```python
from build123d import *

# Parameters (mm, degrees)
CYLINDER026_R     = 1.5
CYLINDER026_DEPTH = 10
CYLINDER025_R     = 1.5
CYLINDER025_DEPTH = 10
CYLINDER024_R     = 1.5
CYLINDER024_DEPTH = 10
CYLINDER027_R     = 1.5
CYLINDER027_DEPTH = 10
BOX022_W          = 15.4
BOX022_H          = 47
BOX022_DEPTH      = 75.8
BOX021_W          = 17.6
BOX021_H          = 51.4
BOX021_DEPTH      = 78


with BuildPart() as obj1:
    # Cylinder026 → Cylinder026 (new body)
    with BuildSketch(Plane(origin=(50, 64.5, 56), x_dir=(0, 0, -1), z_dir=(1, 0, 0))):
        Circle(CYLINDER026_R)
    extrude(amount=CYLINDER026_DEPTH)


with BuildPart() as obj2:
    # Cylinder025 → Cylinder025 (new body)
    with BuildSketch(Plane(origin=(50, 29.5, 50), x_dir=(0, 0, -1), z_dir=(1, 0, 0))):
        Circle(CYLINDER025_R)
    extrude(amount=CYLINDER025_DEPTH)


with BuildPart() as obj3:
    # Cylinder024 → Cylinder024 (new body)
    with BuildSketch(Plane(origin=(50, 29.5, 56), x_dir=(0, 0, -1), z_dir=(1, 0, 0))):
        Circle(CYLINDER024_R)
    extrude(amount=CYLINDER024_DEPTH)


with BuildPart() as obj4:
    # Cylinder027 → Cylinder027 (new body)
    with BuildSketch(Plane(origin=(50, 64.5, 50), x_dir=(0, 0, -1), z_dir=(1, 0, 0))):
        Circle(CYLINDER027_R)
    extrude(amount=CYLINDER027_DEPTH)

    # Fusion015: union obj1, obj2, obj3
    add(obj1.part)
    add(obj2.part)
    add(obj3.part)


with BuildPart() as obj5:
    # Box022 → Box022 (new body)
    with BuildSketch(Plane(origin=(2.2, 2.2, 2.2), x_dir=(1, 0, 0), z_dir=(0, 0, 1))):
        with Locations((7.7, 23.5)):
            Rectangle(BOX022_W, BOX022_H)
    extrude(amount=BOX022_DEPTH)


with BuildPart() as obj6:
    # Box021 → Box021 (new body)
    with BuildSketch(Plane.XY):
        with Locations((8.8, 25.7)):
            Rectangle(BOX021_W, BOX021_H)
    extrude(amount=BOX021_DEPTH)

    # Cut022: cut obj5
    add(obj5.part, mode=Mode.SUBTRACT)


with BuildPart() as obj6_1:
    # Cut022 placement: moved
    add(obj6.part.moved(Location((50.2, 21.3, 41.8))))

    # Cut029: cut obj4
    add(obj4.part, mode=Mode.SUBTRACT)


solid = obj6_1.part
```
For this review, take the finished solid that the model builds, in its own axes (mm). A direction names the side the tool comes from. Round coordinates to 2 decimals unless told otherwise and drop trailing zeros. Write each loop counter-clockwise with the first axis right and the second up, starting at its lowest first coordinate (ties: lowest second). Pieces come first, ordered by that corner, then holes. Notation, with made-up numbers: (-26, 88.25) -> (14, 88.25) arc R9 cw to (14, 94.25) -> close; hole circle Ø6 at (46, -19). An arc over 180 degrees is marked (long way). One line per question, with ' | ' between items. Start each with the question number.
(1) Add section A-A, the plane y = 29.5. Write out the cut boundary in (x, z).
(2) For line 1 along Y through (x, z) = (51.6, 56); line 2 along Z through (x, y) = (51.65, 29.5); line 3 along Y through (x, z) = (61.75, 113), list the stretches that pass through material, from the lowest coordinate up. Write a range as from..to.
(3) Add section B-B, the plane z = 50. Write out the cut boundary in (x, y), plus the area to 3 significant figures.
(4) Add section C-C, the plane x = 56.25. Write out the cut boundary in (y, z).
(5) Tool access review of faces 4 (the face through (60, 47, 44)), 5 (the face through (59, 21.3, 80)): name each direction out of +Z, -Z, +X, -X, +Y, -Y from which nothing blocks a thin tool from reaching the whole face with its end or side.
(6) Add section D-D, the plane y = 42. Write out the cut boundary in (x, z), plus the area to 3 significant figures.
(7) Mouldability with a two-part tool opening along Z and no side actions: class faces 1 (the face through (51.285, 30.765, 55.194)), 2 (the face through (59, 47, 41.8)), 3 (the face through (67.8, 22, 69)) as released by +Z, released by -Z, zero draft, split by the parting line, or undercut.
(8) Insertion check: P1, Ø4, axis at y = 64.5, z = 50, coming from the +X side; P2, Ø4, axis at x = 60, y = 47.5, coming from the +Z side. Each pin has a flat end and moves straight along its axis. Give the tip position at first contact, or say it passes through.
Answer list:
1) outline: (50.2, 41.8) -> (67.8, 41.8) -> (67.8, 44) -> (52.4, 44) -> (52.4, 48.5) -> (50.2, 48.5) -> close; (50.2, 51.5) -> (52.4, 51.5) -> (52.4, 54.5) -> (50.2, 54.5) -> close; (50.2, 57.5) -> (52.4, 57.5) -> (52.4, 119.8) -> (50.2, 119.8) -> close
2) line 1: 21.3..28, 31..63, 66..72.7 | line 2: 41.8..48.5, 51.5..54.5, 57.5..119.8 | line 3: 21.3..23.5, 70.5..72.7
3) outline: (50.2, 21.3) -> (67.8, 21.3) -> (67.8, 23.5) -> (52.4, 23.5) -> (52.4, 28) -> (50.2, 28) -> close; (50.2, 31) -> (52.4, 31) -> (52.4, 63) -> (50.2, 63) -> close; (50.2, 66) -> (52.4, 66) -> (52.4, 70.5) -> (67.8, 70.5) -> (67.8, 72.7) -> (50.2, 72.7) -> close | area: 168 mm²
4) outline: (21.3, 41.8) -> (72.7, 41.8) -> (72.7, 119.8) -> (70.5, 119.8) -> (70.5, 44) -> (23.5, 44) -> (23.5, 119.8) -> (21.3, 119.8) -> close
5) face 4: +Z, +X | face 5: +Z, -Z, +X, -X, -Y
6) outline: (50.2, 41.8) -> (67.8, 41.8) -> (67.8, 44) -> (52.4, 44) -> (52.4, 119.8) -> (50.2, 119.8) -> close | area: 205 mm²
7) face 1: undercut | face 2: released by -Z | face 3: zero draft
8) P1: x = 52.4 | P2: z = 44
